from build123d import *

# Parameters (mm, degrees)
SKETCH1_W               = 127.76
SKETCH1_H               = 85.48
BOSS_EXTRUDE1_DEPTH     = 5
SKETCH3_W               = 2
SKETCH3_H               = 10
CUT_EXTRUDE2_DEPTH      = 1.6
SKETCH4_W               = 2
SKETCH4_H               = 6
CUT_EXTRUDE3_DEPTH      = 95.754317257
MIRROR2_COPY_1_SKETCH_W = 2
MIRROR2_COPY_1_SKETCH_H = 10
MIRROR2_COPY_1_DEPTH    = 1.6
MIRROR2_COPY_2_SKETCH_W = 2
MIRROR2_COPY_2_SKETCH_H = 6
MIRROR2_COPY_2_DEPTH    = 95.754317257
SKETCH6_R               = 12.75
CUT_EXTRUDE4_DEPTH      = 4.4
FILLET1_R               = 1


with BuildPart() as part:
    # Sketch1 → Boss-Extrude1 (new body)
    with BuildSketch(Plane.XY):
        with Locations((9.206235294, -17.469823529)):
            Rectangle(SKETCH1_W, SKETCH1_H)
    extrude(amount=BOSS_EXTRUDE1_DEPTH)

    # Sketch3 → Cut-Extrude2 (cut)
    with BuildSketch(Plane.XY.offset(5)):
        with Locations((-51.673764706, 5.270176471)):
            Rectangle(SKETCH3_W, SKETCH3_H)
    cut_extrude2 = extrude(amount=-CUT_EXTRUDE2_DEPTH, mode=Mode.SUBTRACT)

    # Sketch4 → Cut-Extrude3 (cut, through all)
    with BuildSketch(Plane.XY.offset(3.4)):
        with Locations((-51.673764706, 5.270176471)):
            Rectangle(SKETCH4_W, SKETCH4_H)
    cut_extrude3 = extrude(amount=-CUT_EXTRUDE3_DEPTH, mode=Mode.SUBTRACT)

    # Mirror1: Cut-Extrude2, Cut-Extrude3 across plane
    add(cut_extrude2.mirror(Plane.ZY.offset(-9.206235294)), mode=Mode.SUBTRACT)
    add(cut_extrude3.mirror(Plane.ZY.offset(-9.206235294)), mode=Mode.SUBTRACT)

    # Mirror2: Cut-Extrude2, Cut-Extrude3 across plane
    add(cut_extrude2.mirror(Plane.ZX.offset(-17.469823529)), mode=Mode.SUBTRACT)
    add(cut_extrude3.mirror(Plane.ZX.offset(-17.469823529)), mode=Mode.SUBTRACT)

    # Mirror2 copy 1 sketch → Mirror2 copy 1 (cut)
    with BuildSketch(Plane(origin=(18.412470588, -34.939647059, 5), x_dir=(-1, 0, 0), z_dir=(0, 0, 1))):
        with Locations((-51.673764706, 5.270176471)):
            Rectangle(MIRROR2_COPY_1_SKETCH_W, MIRROR2_COPY_1_SKETCH_H)
    extrude(amount=-MIRROR2_COPY_1_DEPTH, mode=Mode.SUBTRACT)

    # Mirror2 copy 2 sketch → Mirror2 copy 2 (cut, through all)
    with BuildSketch(Plane(origin=(18.412470588, -34.939647059, 3.4), x_dir=(-1, 0, 0), z_dir=(0, 0, 1))):
        with Locations((-51.673764706, 5.270176471)):
            Rectangle(MIRROR2_COPY_2_SKETCH_W, MIRROR2_COPY_2_SKETCH_H)
    extrude(amount=-MIRROR2_COPY_2_DEPTH, mode=Mode.SUBTRACT)

    # Sketch6 → Cut-Extrude4 (cut)
    with BuildSketch(Plane(origin=(0, 0, 0), x_dir=(-1, 0, 0), z_dir=(0, 0, -1))):
        with Locations((-9.206235294, -17.469823529)):
            Circle(SKETCH6_R)
    extrude(amount=-CUT_EXTRUDE4_DEPTH, mode=Mode.SUBTRACT)

    # Fillet1
    fillet1_edges = [part.edges().sort_by_distance(p)[0] for p in [
        (-54.673764706, 25.270176471, 2.5),
        (73.086235294, 25.270176471, 2.5),
        (73.086235294, -60.209823529, 2.5),
        (-54.673764706, -60.209823529, 2.5),
    ]]
    fillet(fillet1_edges, radius=FILLET1_R)


solid = part.part
Can you work these out from the model? Positions are in its coordinate system, mm. A direction names the side the tool comes from. Give positions to 0.01 mm unless a question says otherwise; leave off trailing zeros. Loops run counter-clockwise (first coordinate to the right, second up) from the corner with the lowest first, then second, coordinate; pieces in that order, holes last. Notation, with made-up numbers: (22.5, 4.25) - (46.5, 4.25) arc R20 ccw to (46.5, 31.25) - close; hole circle Ø9 at (50, 28). An arc over 180 degrees is marked (long way). Return JSON: item names as keys, results as strings.
1. We'd pull the mould along Y, two halves only. Please class faces 4 (the face through (8, -60.21, 2)), 5 (the face through (69.086, 5, 3)), 6 (the face through (-50.674, 5, 3)), 7 (the face through (8, -17, 5)): +Y half, -Y half, draft (parallel to the pull), parting line (faces both ways), or undercut.
Output values:
{"face 4": "-Y half", "face 5": "undercut", "face 6": "undercut", "face 7": "draft"}
2. I'm going to push a flat-ended pin straight in: pin 1 Ø5 at (x, y) = (13, -46) entering from -Z. Where does the tip first touch, or does it pass through?
Output values:
{"pin 1": "stops at z = 0"}
3. I want a section at C-C on y = -26.5. Please give me the cut outline in (x, z).
Output values:
{"outline": "(-54.67, 0) - (0.21, 0) - (0.21, 4.4) - (18.21, 4.4) - (18.21, 0) - (73.09, 0) - (73.09, 5) - (-54.67, 5) - close"}
4. If I drill on line 1 (X direction, y = -39, z = 1.25); line 2 (Y direction, x = 9.5, z = 3.9); line 3 (Z direction, x = 18.5, y = -25.5), over which ranges is the centre line in solid material (lowest first)?
Output values:
{"line 1": "x = -54.67 to -52.67, -50.67 to 69.09, 71.09 to 73.09", "line 2": "y = -60.21 to -30.22, -4.72 to 25.27", "line 3": "z = 4.4 to 5"}
5. I want a section at B-B on x = 7.5. Please give me the cut outline in (y, z).
Output values:
{"outline": "(-60.21, 0) - (-30.11, 0) - (-30.11, 4.4) - (-4.83, 4.4) - (-4.83, 0) - (25.27, 0) - (25.27, 5) - (-60.21, 5) - close"}
6. For faces 1 (the face through (-52.674, 5, 3)), 2 (the face through (8, 25.27, 2)), 3 (the face through (9, -17, 4.4)), which set-ups out of +Z, -Z, +X, -X, +Y, -Y let a thin tool reach every point of the face, with its end or its side?
Output values:
{"face 1": "+Z", "face 2": "+Z, -Z, +X, -X, +Y", "face 3": "-Z"}
7. I want a section at A-A on z = 0.95. Please give me the cut outline in (x, y).
Output values:
{"outline": "(-54.67, -59.21) arc R1 ccw to (-53.67, -60.21) - (72.09, -60.21) arc R1 ccw to (73.09, -59.21) - (73.09, 24.27) arc R1 ccw to (72.09, 25.27) - (-53.67, 25.27) arc R1 ccw to (-54.67, 24.27) - close; hole (-52.67, -43.21) - (-50.67, -43.21) - (-50.67, -37.21) - (-52.67, -37.21) - close; hole (-52.67, 2.27) - (-50.67, 2.27) - (-50.67, 8.27) - (-52.67, 8.27) - close; hole circle Ø25.5 at (9.21, -17.47); hole (69.09, -43.21) - (71.09, -43.21) - (71.09, -37.21) - (69.09, -37.21) - close; hole (69.09, 2.27) - (71.09, 2.27) - (71.09, 8.27) - (69.09, 8.27) - close"}
